from build123d import *

# Parameters (mm, degrees)
SKETCH1_W           = 160
SKETCH1_H           = 110
SKETCH1_R           = 6.5
SKETCH1_R_2         = 7.5
BOSS_EXTRUDE1_DEPTH = 10
SKETCH2_R           = 2
CUT_EXTRUDE1_DEPTH  = 5


with BuildPart() as part:
    # Sketch1 → Boss-Extrude1 (new body)
    with BuildSketch(Plane(origin=(0, 0, 0), x_dir=(1, 0, 0), z_dir=(0, 1, 0))):
        Rectangle(SKETCH1_W, SKETCH1_H)
        with Locations(Location((-55, 0, 0), (0, 0, 270))):
            Circle(SKETCH1_R, mode=Mode.SUBTRACT)
        with Locations(Location((55, 0, 0), (0, 0, 90))):
            Circle(SKETCH1_R, mode=Mode.SUBTRACT)
        with Locations(Location((0, 0, 0), (0, 0, 270))):
            Circle(SKETCH1_R_2, mode=Mode.SUBTRACT)
        with BuildLine():
            Line((-25, 31.224989992), (-25, 27.276363394))
            ThreePointArc((-25, 27.276363394), (0, 37), (25, 27.276363394))
            Line((25, 27.276363394), (25, 31.224989992))
            ThreePointArc((25, 31.224989992), (0, 40), (-25, 31.224989992))
        make_face(mode=Mode.SUBTRACT)
        with BuildLine():
            Line((-25, -27.276363394), (-25, -31.224989992))
            ThreePointArc((-25, -31.224989992), (0, -40), (25, -31.224989992))
            Line((25, -31.224989992), (25, -27.276363394))
            ThreePointArc((25, -27.276363394), (0, -37), (-25, -27.276363394))
        make_face(mode=Mode.SUBTRACT)
    extrude(amount=BOSS_EXTRUDE1_DEPTH)

    # Sketch2 → Cut-Extrude1 (cut)
    with BuildSketch(Plane(origin=(0, 10, 0), x_dir=(1, 0, 0), z_dir=(0, 1, 0))):
        with Locations(Location((-12, 0, 0), (0, 0, 270))):
            Circle(SKETCH2_R)
        with Locations(Location((12, 0, 0), (0, 0, 90))):
            Circle(SKETCH2_R)
    extrude(amount=-CUT_EXTRUDE1_DEPTH, mode=Mode.SUBTRACT)


solid = part.part
Read the model definition and answer for the solid it produces. Units are mm, in the model's axes. A direction names the side the tool comes from. Round coordinates to 2 decimals unless told otherwise and drop trailing zeros. Loops run counter-clockwise (first coordinate to the right, second up) from the corner with the lowest first, then second, coordinate; pieces in that order, holes last.
Q1. Determine the mould class of faces 1 (the face through (-1, 5, -55)), 2 (the face through (10, 8, 0)), 3 (the face through (-80, 5, 1)) for opening direction X: released by +X, released by -X, zero draft, split by the parting line, or undercut.
Q2. This flat-tipped pin is pushed along its axis until it touches: pin 1 (1.2 mm diameter, centred on x = -11.5, z = 0.5, fed in from +Y). Where does it stop, or does it pass through?
Q3. Section C-C on z = 0 is taken. Write down the section's boundary in (x, y), and give its area (3 significant figures).
Q4. Which of the six approach directions +Z, -Z, +X, -X, +Y, -Y give full straight-line access (tool end or side, diameter ignored) to faces 4 (the face through (0, 5, 40)), 5 (the face through (80, 5, 1)), 6 (the face through (-10, 8, 0))?
Q5. Section B-B on y = 7 is taken. Write down the section's boundary in (x, z), and give its area (3 significant figures).
Q6. Section A-A on x = 0 is taken. Write down the section's boundary in (y, z), and give its area (3 significant figures).
Q7. Section D-D on x = 55 is taken. Write down the section's boundary in (y, z), and give its area (3 significant figures).
Q8. Consider probe 1 along X at (y, z) = (3.75, 0); probe 2 along X at (y, z) = (6.75, 0); probe 3 along Z at (x, y) = (12, 7.75). Determine where each line is inside the solid, lowest interval first.
Output:
1. face 1: zero draft
1. face 2: undercut
1. face 3: released by -X
2. pin 1: stops at y = 5
3. outline: (-80, 0) - (-61.5, 0) - (-61.5, 10) - (-80, 10) - close; (-48.5, 0) - (-7.5, 0) - (-7.5, 10) - (-10, 10) - (-10, 5) - (-14, 5) - (-14, 10) - (-48.5, 10) - close; (7.5, 0) - (48.5, 0) - (48.5, 10) - (14, 10) - (14, 5) - (10, 5) - (10, 10) - (7.5, 10) - close; (61.5, 0) - (80, 0) - (80, 10) - (61.5, 10) - close
3. area: 1,150 mm2
4. face 4: +Y, -Y
4. face 5: +Z, -Z, +X, +Y, -Y
4. face 6: +Y
5. outline: (-80, -55) - (80, -55) - (80, 55) - (-80, 55) - close; hole circle Ø13 at (-55, 0); hole (-25, -31.22) arc R40 ccw to (25, -31.22) - (25, -27.28) arc R37 cw to (-25, -27.28) - close; hole (-25, 27.28) arc R37 cw to (25, 27.28) - (25, 31.22) arc R40 ccw to (-25, 31.22) - close; hole circle Ø4 at (-12, 0); hole circle Ø15 at (0, 0); hole circle Ø4 at (12, 0); hole circle Ø13 at (55, 0)
5. area: 16,800 mm2
6. outline: (0, -55) - (10, -55) - (10, -40) - (0, -40) - close; (0, -37) - (10, -37) - (10, -7.5) - (0, -7.5) - close; (0, 7.5) - (10, 7.5) - (10, 37) - (0, 37) - close; (0, 40) - (10, 40) - (10, 55) - (0, 55) - close
6. area: 890 mm2
7. outline: (0, -55) - (10, -55) - (10, -6.5) - (0, -6.5) - close; (0, 6.5) - (10, 6.5) - (10, 55) - (0, 55) - close
7. area: 970 mm2
8. probe 1: x = -80 to -61.5, -48.5 to -7.5, 7.5 to 48.5, 61.5 to 80
8. probe 2: x = -80 to -61.5, -48.5 to -14, -10 to -7.5, 7.5 to 10, 14 to 48.5, 61.5 to 80
8. probe 3: z = -55 to -38.16, -35 to -2, 2 to 35, 38.16 to 55
